```python
from build123d import *

# Parameters (mm, degrees)
F0_R     = 1.5875
F1_DEPTH = 17.78


with BuildPart() as f1:
    # F0 (on Front) → F1 (new body)
    with BuildSketch(Plane.XZ):
        with BuildLine():
            ThreePointArc((-46.1619771098, 70.2782855404), (-43.8554341456, 62.7874652309), (-36.7116841456, 59.5626605404))
            ThreePointArc((-36.7116841456, 59.5626605404), (-29.9764920548, 62.3524684496), (-27.1866841456, 69.0876605404))
            ThreePointArc((-27.1866841456, 69.0876605404), (-36.1152009036, 78.5939654346), (-46.1619771098, 70.2782855404))
        make_face()
        with BuildLine():
            ThreePointArc((-33.5366841456, 69.0876605404), (-34.4666201153, 66.8425965101), (-36.7116841456, 65.9126605404))
            ThreePointArc((-36.7116841456, 65.9126605404), (-38.9567481759, 71.3327245707), (-33.5366841456, 69.0876605404))
        make_face(mode=Mode.SUBTRACT)
        with BuildLine():
            Line((-36.7116841456, 34.1626605404), (-36.7116841456, 59.5626605404))
            ThreePointArc((-36.7116841456, 59.5626605404), (-43.8554341456, 62.7874652309), (-46.1619771098, 70.2782855404))
            Line((-46.1619771098, 70.2782855404), (-52.4621724193, 20.2720355404))
            ThreePointArc((-52.4621724193, 20.2720355404), (-47.2120096614, 30.1939105404), (-36.7116841456, 34.1626605404))
        make_face()
        with Locations((-40.8617444336, 54.8128605404)):
            Circle(F0_R, mode=Mode.SUBTRACT)
        with BuildLine():
            ThreePointArc((-27.1866841456, 69.0876605404), (-29.9764920548, 62.3524684496), (-36.7116841456, 59.5626605404))
            Line((-36.7116841456, 59.5626605404), (-36.7116841456, 34.1626605404))
            ThreePointArc((-36.7116841456, 34.1626605404), (-26.2204012908, 30.2018793171), (-20.9642272409, 20.2959498708))
            Line((-20.9642272409, 20.2959498708), (-27.1866841456, 69.0876605404))
        make_face()
        with BuildLine():
            Line((-36.7116841456, 21.4626605404), (-36.7116841456, 34.1626605404))
            ThreePointArc((-36.7116841456, 34.1626605404), (-47.2120096614, 30.1939105404), (-52.4621724193, 20.2720355404))
            ThreePointArc((-52.4621724193, 20.2720355404), (-52.585427961, 18.4873660271), (-52.5071097097, 16.7001605404))
            ThreePointArc((-52.5071097097, 16.7001605404), (-47.3609578884, 6.5144454421), (-36.7116841456, 2.4126605404))
            Line((-36.7116841456, 2.4126605404), (-36.7116841456, 15.1126605404))
            ThreePointArc((-36.7116841456, 15.1126605404), (-39.8866841456, 18.2876605404), (-36.7116841456, 21.4626605404))
        make_face()
        with BuildLine():
            ThreePointArc((-20.9642272409, 20.2959498708), (-26.2204012908, 30.2018793171), (-36.7116841456, 34.1626605404))
            Line((-36.7116841456, 34.1626605404), (-36.7116841456, 21.4626605404))
            ThreePointArc((-36.7116841456, 21.4626605404), (-34.4666201153, 20.5327245707), (-33.5366841456, 18.2876605404))
            ThreePointArc((-33.5366841456, 18.2876605404), (-34.4666201153, 16.0425965101), (-36.7116841456, 15.1126605404))
            Line((-36.7116841456, 15.1126605404), (-36.7116841456, 2.4126605404))
            ThreePointArc((-36.7116841456, 2.4126605404), (-26.0624104027, 6.5144454421), (-20.9162585815, 16.7001605404))
            ThreePointArc((-20.9162585815, 16.7001605404), (-20.856590235, 17.4929139863), (-20.8366841456, 18.2876605404))
            ThreePointArc((-20.8366841456, 18.2876605404), (-20.868602006, 19.29382818), (-20.9642272409, 20.2959498708))
        make_face()
        with BuildLine():
            ThreePointArc((-36.7116841456, 2.4126605404), (-47.3609578884, 6.5144454421), (-52.5071097097, 16.7001605404))
            Line((-52.5071097097, 16.7001605404), (-46.188939484, -46.1648394596))
            ThreePointArc((-46.188939484, -46.1648394596), (-43.7756132045, -38.8227752139), (-36.7116841456, -35.6873394596))
            Line((-36.7116841456, -35.6873394596), (-36.7116841456, 2.4126605404))
        make_face()
        with BuildLine():
            ThreePointArc((-20.9162585815, 16.7001605404), (-26.0624104027, 6.5144454421), (-36.7116841456, 2.4126605404))
            Line((-36.7116841456, 2.4126605404), (-36.7116841456, -35.6873394596))
            ThreePointArc((-36.7116841456, -35.6873394596), (-29.9764920548, -38.4771473688), (-27.1866841456, -45.2123394596))
            Line((-27.1866841456, -45.2123394596), (-0.1991841456, -45.2123394596))
            ThreePointArc((-0.1991841456, -45.2123394596), (2.2264053697, -39.5007066757), (8.020721129, -37.279864845))
            Line((8.020721129, -37.279864845), (-17.7433562776, -36.362633879))
            ThreePointArc((-17.7433562776, -36.362633879), (-23.4504801631, -33.6448765637), (-25.3708482771, -27.622447305))
            Line((-25.3708482771, -27.622447305), (-20.9162585815, 16.7001605404))
        make_face()
        with BuildLine():
            ThreePointArc((-36.7116841456, -35.6873394596), (-43.7756132045, -38.8227752139), (-46.188939484, -46.1648394596))
            ThreePointArc((-46.188939484, -46.1648394596), (-42.9740675272, -52.3892593687), (-36.3715055742, -54.7312629039))
            ThreePointArc((-36.3715055742, -54.7312629039), (-29.8572758599, -51.8261667973), (-27.1866841456, -45.2123394596))
            Line((-27.1866841456, -45.2123394596), (-33.5366841456, -45.2123394596))
            ThreePointArc((-33.5366841456, -45.2123394596), (-38.9567481759, -47.4574034899), (-36.7116841456, -42.0373394596))
            Line((-36.7116841456, -42.0373394596), (-36.7116841456, -35.6873394596))
        make_face()
        with BuildLine():
            ThreePointArc((-27.1866841456, -45.2123394596), (-29.9764920548, -38.4771473688), (-36.7116841456, -35.6873394596))
            Line((-36.7116841456, -35.6873394596), (-36.7116841456, -42.0373394596))
            ThreePointArc((-36.7116841456, -42.0373394596), (-34.4666201153, -42.9672754293), (-33.5366841456, -45.2123394596))
            Line((-33.5366841456, -45.2123394596), (-27.1866841456, -45.2123394596))
        make_face()
        with BuildLine():
            ThreePointArc((-0.1991841456, -45.2123394596), (2.226793073, -50.9243463643), (8.0217979973, -53.1447756632))
            ThreePointArc((8.0217979973, -53.1447756632), (13.4503227591, -50.723862241), (15.6758158544, -45.2123394596))
            ThreePointArc((15.6758158544, -45.2123394596), (13.4499486383, -39.7004289749), (8.020721129, -37.279864845))
            ThreePointArc((8.020721129, -37.279864845), (2.2264053697, -39.5007066757), (-0.1991841456, -45.2123394596))
        make_face()
        with BuildLine():
            ThreePointArc((10.9133158544, -45.2123394596), (7.7383158544, -48.3873394596), (4.5633158544, -45.2123394596))
            ThreePointArc((4.5633158544, -45.2123394596), (7.7383158544, -42.0373394596), (10.9133158544, -45.2123394596))
        make_face(mode=Mode.SUBTRACT)
        with BuildLine():
            ThreePointArc((-27.1866841456, -45.2123394596), (-29.8572758599, -51.8261667973), (-36.3715055742, -54.7312629039))
            Line((-36.3715055742, -54.7312629039), (8.0217979973, -53.1447756632))
            ThreePointArc((8.0217979973, -53.1447756632), (2.226793073, -50.9243463643), (-0.1991841456, -45.2123394596))
            Line((-0.1991841456, -45.2123394596), (-27.1866841456, -45.2123394596))
        make_face()
    extrude(amount=F1_DEPTH)


solid = f1.part
```
Work out the finished part from the listing and answer in its coordinate system (mm). A direction names the side the tool comes from. Round coordinates to 2 decimals unless told otherwise and drop trailing zeros. Write each loop counter-clockwise with the first axis right and the second up, starting at its lowest first coordinate (ties: lowest second). Pieces come first, ordered by that corner, then holes. Notation, with made-up numbers: (17, -33) -> (52, -33) arc R33 ccw to (52, 6) -> close; hole circle Ø2 at (88, 47.5). An arc over 180 degrees is marked (long way). Write each question's results on one line, items separated by ' | '.
Q1. Section C-C, the plane y = -3.75 is taken. Give the number of separate pieces and of enclosed holes in the cut face, then the cut area to 3 significant figures.
Data:
separate pieces: 1 | enclosed holes: 5 | area: 3,800 mm^2
Q2. Flat-ended cylindrical pins translate along their axes: P1, Ø1, axis at y = -7, z = 40, coming from the -X side; P2, Ø10, axis at y = -7, z = -33, coming from the -X side; P3, Ø10, axis at x = -23.5, y = -9.5, coming from the -Z side; P4, Ø8.5, axis at x = -36.71, z = -45.21, coming from the +Y side. Find the tip coordinate at first contact, or state that the pin passes through.
Data:
P1: x = -50.04 | P2: x = -48.01 | P3: z = -54.45 | P4: y = 0
Q3. Section A-A, the plane x = -23.5 is taken. Write down the section's boundary in (y, z).
Data:
outline: (-17.78, -54.27) -> (0, -54.27) -> (0, -33.59) -> (-17.78, -33.59) -> close; (-17.78, -9.01) -> (0, -9.01) -> (0, 40.18) -> (-17.78, 40.18) -> close
Q4. Determine the mould class of faces 1 (the flat face through (-24.03, -8.77, 44.35)), 2 (the cylindrical face through (-23.4, -8.8, -33.7)), 3 (the cylindrical face through (-52.585, -8.766, 18.512)), 4 (the cylindrical face through (-43.05, -8.77, -52.32)) for opening direction Z: released by +Z, released by -Z, zero draft, split by the parting line, or undercut.
Data:
face 1: released by +Z | face 2: undercut | face 3: split by the parting line | face 4: released by -Z
Q5. Straight lines are drawn through the part: line 1 along Z through (x, y) = (-36.5, -12.25); line 2 along Z through (x, y) = (-35.5, -10.5); line 3 along X through (y, z) = (-15.75, -45). For each, find the intervals that lie inside material, in ascending order. Write a range as [from, to].
Data:
line 1: [-54.73, -48.38], [-42.04, 15.12], [21.46, 65.92], [72.26, 78.61] | line 2: [-54.7, -48.15], [-42.28, 15.35], [21.22, 66.15], [72.02, 78.54] | line 3: [-46.31, -39.88], [-33.54, 4.57], [10.91, 15.67]
Q6. Which of the six approach directions +Z, -Z, +X, -X, +Y, -Y give full straight-line access (tool end or side, diameter ignored) to faces 5 (the flat face through (-49.268, -8.766, 45.625)), 6 (the flat face through (-23.175, -8.766, -5.771))?
Data:
face 5: +Z, -X, +Y, -Y | face 6: +X, +Y, -Y
Q7. Section D-D, the plane z = -6 is taken. Write down the section's boundary in (x, y).
Data:
outline: (-50.23, -17.78) -> (-23.2, -17.78) -> (-23.2, 0) -> (-50.23, 0) -> close
Q8. Section B-B, the plane x = -38 is taken. Write down the section's boundary in (y, z).
Data:
outline: (-17.78, -54.65) -> (0, -54.65) -> (0, -48.11) -> (-17.78, -48.11) -> close; (-17.78, -42.31) -> (0, -42.31) -> (0, 15.39) -> (-17.78, 15.39) -> close; (-17.78, 21.19) -> (0, 21.19) -> (0, 66.19) -> (-17.78, 66.19) -> close; (-17.78, 71.99) -> (0, 71.99) -> (0, 78.53) -> (-17.78, 78.53) -> close
